Autodesk Inventor part; units mm, degrees
ref_plane "YZ Plane" through (0, 0, 0) normal (1, 0, 0) x (0, 1, 0)
ref_plane "XZ Plane" through (0, 0, 0) normal (0, 1, 0) x (-1, 0, 0)
ref_plane "XY Plane" through (0, 0, 0) normal (0, 0, 1) x (1, 0, 0)
sketch "Sketch1" plane through (0, 0, 0) normal (0, 0, 1) x (1, 0, 0)
  line L0 (0, 0) -> (0, 8.5511) construction
  line L1 (17.5, 0) -> (17.5, 2)
  line L2 (17.5, 2) -> (20.5, 2)
  line L3 (20.5, 2) -> (20.5, 4)
  line L4 (20.5, 4) -> (20, 4)
  line L5 (20, 4) -> (20, 10)
  line L6 (20, 10) -> (22.5, 10)
  line L7 (22.5, 10) -> (22.5, 0)
  line L8 (22.5, 0) -> (17.5, 0)
  dimension "d0" = 35
  dimension "d1" = 2
  dimension "d2" = 2
  dimension "d3" = 40
  dimension "d4" = 0.5
  dimension "d5" = 6
  dimension "d6" = 45
revolve "Revolution1" add sketch "Sketch1" angle 360 about axis through (0, 0, 0) along (0, 1, 0)
thread "Thread1"
properties part number "004" material "Brass, Soft Yellow"
Geometry: final body of the model. Coordinates: model frame, mm. A direction names the side the tool comes from. Round coordinates to 2 decimals unless told otherwise and drop trailing zeros. Order: outer loops, then holes, each group sorted by start corner. A loop starts at its lowest first (then second) coordinate and runs counter-clockwise, first axis right, second up. Notation, with made-up numbers: M 41.25,15 L 59.25,15 A21 ccw 59.25,51 Z; hole C -21,87 d6. An arc over 180 degrees is marked long. Use one line per item in the form item = value. Start each with the question number.
Q1. Cut plane C-C (y = 1). Return loops of the section in (x, z), and give its area (3 significant figures).
Q2. Mould query, pull axis Z, two halves, no side actions, for faces 4 (the face through (12, 0, 13)), 5 (the face through (10.382, 4.93, -19.961)), 6 (the face through (18.1, 4, 9)). Classes: +Z half, -Z half, draft (parallel to the pull), parting line (faces both ways), or undercut.
Q3. Cut plane A-A (x = 0). Return loops of the section in (y, z), and give its area (3 significant figures).
Q4. Cut plane B-B (z = 0). Return loops of the section in (x, y).
Q5. Access query for faces 1 (the face through (-13.887, 1.014, 10.648)), 2 (the face through (15.1, 2, -9.2)), 3 (the face through (-4.336, 7.042, 19.524)). Directions: +Z, -Z, +X, -X, +Y, -Y. A direction counts if a zero-diameter tool reaches every point of the face in a straight line with its end or side. Return the directions, or none.
Q6. Pin query (flat end, axial travel): pin 1 Ø1 at (y, z) = (2.5, -9) entering from +X; pin 2 Ø1 at (x, y) = (-11.5, 8.5) entering from +Z; pin 3 Ø3 at (x, y) = (11, 5.5) entering from +Z. Return the tip coordinate at first contact, or that it passes through.
Q7. Material intervals for line 1 (Z direction, x = 0, y = 2.8); line 2 (X direction, y = 5.6, z = 0); line 3 (Y direction, x = 12.5, z = -16), sorted ascending. Write a range as [from, to].
Q8. Cut plane D-D (y = 7). Return loops of the section in (x, z).
Geometry results:
q1.outline = C 0,0 d45; hole C 0,0 d35
q1.area = 628 mm^2
q2.face_4 = draft
q2.face_5 = parting line
q2.face_6 = undercut
q3.outline = M 0,-22.5 L 10,-22.5 L 10,-20 L 4,-20 L 4,-20.5 L 2,-20.5 L 2,-17.5 L 0,-17.5 Z; M 0,17.5 L 2,17.5 L 2,20.5 L 4,20.5 L 4,20 L 10,20 L 10,22.5 L 0,22.5 Z
q3.area = 58.0 mm^2
q4.outline = M -22.5,0 L -17.5,0 L -17.5,2 L -20.5,2 L -20.5,4 L -20,4 L -20,10 L -22.5,10 Z; M 17.5,0 L 22.5,0 L 22.5,10 L 20,10 L 20,4 L 20.5,4 L 20.5,2 L 17.5,2 Z
q5.face_1 = +Y, -Y
q5.face_2 = none
q5.face_3 = +Y
q6.pin_1 = 20.83
q6.pin_2 = 19.63
q6.pin_3 = 20.4
q7.line_1 = [-22.5, -20.5], [20.5, 22.5]
q7.line_2 = [-22.5, -20], [20, 22.5]
q7.line_3 = [0, 2], [4, 10]
q8.outline = C 0,0 d45; hole C 0,0 d40
